Autodesk Inventor part; units mm, degrees
ref_plane "YZ Plane" through (0, 0, 0) normal (1, 0, 0) x (0, 1, 0)
ref_plane "XZ Plane" through (0, 0, 0) normal (0, 1, 0) x (-1, 0, 0)
ref_plane "XY Plane" through (0, 0, 0) normal (0, 0, 1) x (1, 0, 0)
sketch "Эскиз1" plane through (0, 0, 0) normal (0, 1, 0) x (-1, 0, 0)
  line L0 (0, 0) -> (40, 0)
  line L1 (40, 0) -> (40, -20)
  line L2 (40, -20) -> (0, -20)
  line L3 (0, -20) -> (0, 0)
  line L4 (37, -3) -> (3, -3)
  line L5 (3, -3) -> (3, -17)
  line L6 (3, -17) -> (37, -17)
  line L7 (37, -17) -> (37, -3)
  dimension "d0" = 20
  dimension "d1" = 40
  dimension "d2" = 3
extrude "Выдавливание1" add sketch "Эскиз1" along normal blind 400
sketch "Эскиз2" plane through (-40, 0, 0) normal (0, 0, 1) x (1, 0, 0)
  line L0 (3, 0) -> (3, 400)
  line L1 (0, 400) -> (40, 400)
  line L2 (20, 819.3664) -> (20, 691.613)
  line L3 (3, 0) -> (37, 0)
  line L4 (37, 0) -> (37, 400)
  line L5 (3, 400) -> (37, 400)
  line L6 (3, 0) -> (3, 400)
  line L7 (37, 0) -> (37, 400)
  spline S0 degree 4 poles (37, 400) (28.1429, 400) (6.6723, 373.0542) (29.5104, 351.5723) (31.0092, 323.4583) (3, 323.4583) knots 0 0 0 0 0 0.490634 1 1 1 1 1
  line L8 (22.2784, 323.4583) -> (-16.2784, 323.4583) construction
  arc A0 (-12.0901, 325.0339) -> (18.0901, 325.0339) centre (3, 396.5064) ccw construction
  line L9 (44.0036, 400) -> (29.9964, 400) construction
  arc A1 (41.5725, 398.5449) -> (32.4275, 398.5449) centre (37, 392.0879) ccw construction
  line L10 (3, 323.4583) -> (0, 323.4583)
  line L11 (0, 0) -> (0, 400)
  line L12 (0, 323.4583) -> (0, 400)
  point P0 (40, 0)
  point P1 (20, 381.1712)
  point P2 (25.6195, 346.1519)
extrude "Выдавливание2" cut sketch "Эскиз2" against normal through all contours L10 L11 L1 L0 | L0 L1 S0
equation "\"d0\" = width_profile_tibea"
equation "\"d1\" = hight_profile_tibea"
equation "\"d2\" = thickness_profile_tibea"
equation "\"d3\" = length_thorn_tibia"
equation "\"d_main_shaft\" = 15"
equation "\"width_profile_tibea\" = 20"
equation "\"hight_profile_tibea\" = 40"
equation "\"thickness_profile_tibea\" = 3"
equation "\"tolerance_plazma\" = 0.1"
equation "\"d_main_screw_holes\" = 6.1"
equation "\"length_thorn_tibia\" = 400"
equation "\"thickness_steel\" = 3"
equation "\"hight_shaft_shift\" = 37"
equation "\"thickness_profile_femur\" = 3"
equation "\"width_shaft_shift\" = 35"
equation "\"width_flattened_surface\" = 12"
properties part number "tibea_profile" material "Алюминий"
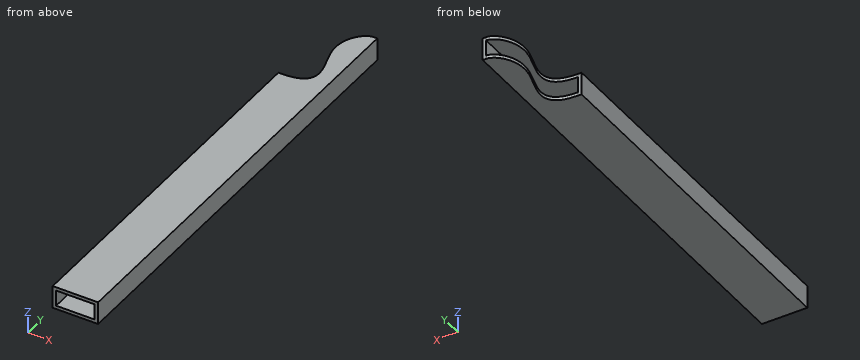
For this review, take the finished solid that the model builds, in its own axes (mm). Coordinates: 2 decimals unless noted, no trailing zeros. Order: outer loops, then holes, each group sorted by start corner. A loop starts at its lowest first (then second) coordinate and runs counter-clockwise, first axis right, second up. Notation, with made-up numbers: (-29, -30.75) - (-4, -30.75) arc R16 cw to (-4, -20.75) - close; hole circle Ø10 at (-8, 23.25). An arc over 180 degrees is marked (long way). Answer as a JSON object with one key per item and string values. Group by question number.
1. For probe 1 along X at (y, z) = (92.5, -12.5); probe 2 along Z at (x, y) = (-7.5, 256), list the stretches that pass through material, from the lowest coordinate up.
2. We need section B-B on y = 265. State the section outline as (x, z) points.
3. Clearance check with flat-ended pins moving along their axes: P1, Ø12, axis at x = -9.5, z = -15, coming from the +Y side; P2, Ø2.5, axis at x = -39, z = -14, coming from the +Y side. State where each tip first meets the part, or that it passes through.
4. We need section C-C on x = -20. Give the number of separate pieces and of enclosed holes in the cut face, then the cut area to 3 significant figures.
5. We need section A-A on z = -11.25. State the section outline as (x, y) points.
Final values:
{
 "1": {"probe 1": "-40 to -37, -3 to 0", "probe 2": "-20 to -17, -3 to 0"},
 "2": {"outline": "(-40, -20) - (0, -20) - (0, 0) - (-40, 0) - close; hole (-37, -17) - (-3, -17) - (-3, -3) - (-37, -3) - close"},
 "3": {"P1": "y = 399.96", "P2": "y = 323.46"},
 "4": {"separate pieces": "4", "enclosed holes": "0", "area": "2,050 mm²"},
 "5": {"outline": "(-40, 0) - (-37, 0) - (-37, 323.46) - (-40, 323.46) - close; (-3, 0) - (0, 0) - (0, 400) - (-3, 400) - close"}
}
